Could you check a few things on this model? Use its own coordinates, in mm. Face numbers are marked on the shaded views. A direction names the side the tool comes from. Round coordinates to 2 decimals unless told otherwise and drop trailing zeros. Write each loop counter-clockwise with the first axis right and the second up, starting at its lowest first coordinate (ties: lowest second). Pieces come first, ordered by that corner, then holes. Notation, with made-up numbers: (-32.75, 24.5) -> (-7.75, 24.5) arc R20 ccw to (-7.75, 52.5) -> close; hole circle Ø5 at (23.25, 8). An arc over 180 degrees is marked (long way). Answer in a Markdown table with one row per item.
from build123d import *

# Parameters (mm, degrees)
SKETCH049_W  = 400
SKETCH049_H  = 60
PAD_DEPTH    = 300
SKETCH050_W  = 412
SKETCH050_H  = 50
PAD001_DEPTH = 306
SKETCH051_W  = 512
SKETCH051_H  = 712
PAD002_DEPTH = 6


with BuildPart() as body:
    # Sketch049 → Pad (new body, symmetric)
    with BuildSketch(Plane.XZ):
        with Locations((0, 30)):
            Rectangle(SKETCH049_W, SKETCH049_H)
    extrude(amount=PAD_DEPTH, both=True)


with BuildPart() as cut006:
    # Sketch050 → Pad001 (new body, symmetric)
    with BuildSketch(Plane.XZ):
        with Locations((0, 25)):
            Rectangle(SKETCH050_W, SKETCH050_H)
    extrude(amount=PAD001_DEPTH, both=True)

    # Sketch051 (on Face3 of Pad001) → Pad002 (join)
    with BuildSketch(Plane(origin=(0, 0, 50), x_dir=(-1, 0, 0), z_dir=(0, 0, 1))):
        Rectangle(SKETCH051_W, SKETCH051_H)
    extrude(amount=PAD002_DEPTH)

    # Cut006: cut Body
    add(body.part, mode=Mode.SUBTRACT)


solid = cut006.part
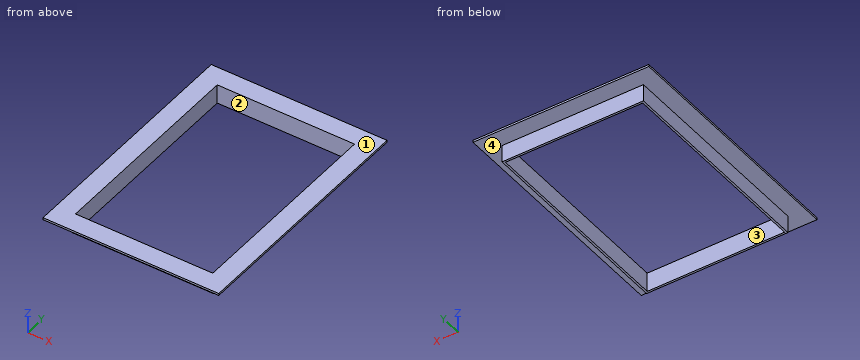
1) Imagine slicing it at C-C, the plane z = 41.5. Please give me the cut outline in (x, y).
Findings:
| item | result |
|---|---|
| outline | (-206, -306) -> (206, -306) -> (206, 306) -> (-206, 306) -> close; hole (-200, -300) -> (200, -300) -> (200, 300) -> (-200, 300) -> close |
2) Imagine slicing it at B-B, the plane y = 118. Please give me the cut outline in (x, z), plus the area to 3 significant figures.
Findings:
| item | result |
|---|---|
| outline | (-256, 50) -> (-206, 50) -> (-206, 0) -> (-200, 0) -> (-200, 56) -> (-256, 56) -> close; (200, 0) -> (206, 0) -> (206, 50) -> (256, 50) -> (256, 56) -> (200, 56) -> close |
| area | 1,270 mm^2 |
3) For the marked faces 1 and 2, which set-ups out of +Z, -Z, +X, -X, +Y, -Y let a thin tool reach every point of the face, with its end or its side?
Findings:
| item | result |
|---|---|
| face 1 | +Z, +X, -X, +Y, -Y |
| face 2 | +Z, -Z |
4) Thinking about a two-plate mould opening in Y: for the marked faces 3 and 4, which applies, +Y half, -Y half, draft (parallel to the pull), parting line (faces both ways), or undercut?
Findings:
| item | result |
|---|---|
| face 3 | undercut |
| face 4 | draft |
5) For pin 1 (3 mm diameter, centred on y = -262.5, z = 48, fed in from +X); pin 2 (2 mm diameter, centred on y = -135.5, z = 45.5, fed in from -X); pin 3 (1 mm diameter, centred on x = 173, z = 9.5, fed in from -Y), each with a flat end and sliding along its axis, tell me the tip position at first contact or that it passes through.
Findings:
| item | result |
|---|---|
| pin 1 | stops at x = 206 |
| pin 2 | stops at x = -206 |
| pin 3 | stops at y = -306 |
6) Please list where these lines run through material, in increasing order: line 1 (Y direction, x = 172, z = 38.5); line 2 (Y direction, x = 20.5, z = 52); line 3 (X direction, y = -18.5, z = 23.5).
Findings:
| item | result |
|---|---|
| line 1 | y = -306 to -300, 300 to 306 |
| line 2 | y = -356 to -300, 300 to 356 |
| line 3 | x = -206 to -200, 200 to 206 |
7) Imagine slicing it at A-A, the plane x = -41. Please give me the cut outline in (y, z), plus the area to 3 significant figures.
Findings:
| item | result |
|---|---|
| outline | (-356, 50) -> (-306, 50) -> (-306, 0) -> (-300, 0) -> (-300, 56) -> (-356, 56) -> close; (300, 0) -> (306, 0) -> (306, 50) -> (356, 50) -> (356, 56) -> (300, 56) -> close |
| area | 1,270 mm^2 |
